Source: CAD feature listing. Evaluate the final solid. Frame: model axes, mm. Face numbers are marked on the shaded views. Round coordinates to 2 decimals unless told otherwise and drop trailing zeros. Loops run counter-clockwise (first coordinate to the right, second up) from the corner with the lowest first, then second, coordinate; pieces in that order, holes last.
(1) Section C-C, the plane y = 0. Return the cut outline in (x, z), plus the area to 3 significant figures.
(2) Section B-B, the plane x = -20. Return the cut outline in (y, z), plus the area to 3 significant figures.
(3) Material intervals for probe 1 along X at (y, z) = (-3.75, -6.35); probe 2 along Z at (x, y) = (4, 1); probe 3 along X at (y, z) = (-0.25, -2), sorted ascending.
(4) Section D-D, the plane x = 35. Return the cut outline in (y, z), plus the area to 3 significant figures.
(5) Section A-A, the plane z = -6.35. Return the cut outline in (x, y).
(6) First-contact query: pin 1 Ø3 at (x, y) = (-35, 0) entering from -Z; pin 2 Ø4 at (x, y) = (-14.5, 2.5) entering from +Z. Flat tips, straight axial feed; report the tip coordinate or a pass-through.
(7) Mould query, pull axis Z, two halves, no side actions, for the marked faces 1, 2 and 3. Classes: pulls with the +Z half, pulls with the -Z half, needs draft (parallel to the pull), parting line crosses it, or undercut.
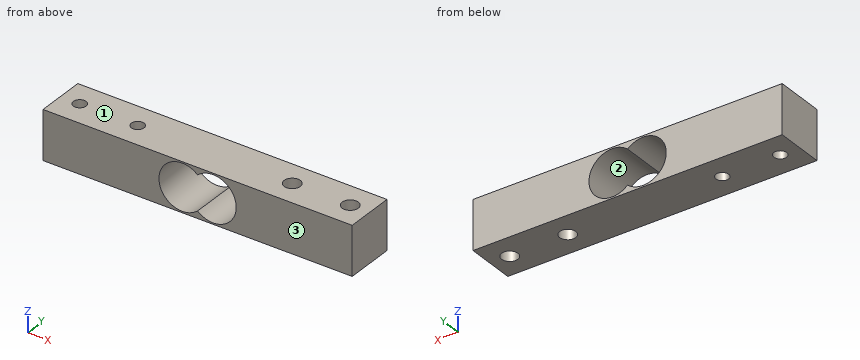
```python
from build123d import *

# Parameters (mm, degrees)
SKETCH1_W               = 80
SKETCH1_H               = 12.7
BOSS_EXTRUDE1_DEPTH     = 12.7
TAP_DRILL_FOR_M5_TAP1_D = 4.2
TAP_DRILL_FOR_M4_TAP1_D = 3.3
SKETCH6_R               = 6
CUT_EXTRUDE1_DEPTH      = 44.847234804


with BuildPart() as part:
    # Sketch1 → Boss-Extrude1 (new body)
    with BuildSketch(Plane.XY):
        Rectangle(SKETCH1_W, SKETCH1_H)
    extrude(amount=-BOSS_EXTRUDE1_DEPTH)

    # Tap Drill for M5 Tap1 (through all)
    with Locations(Plane.XY):
        with Locations((20, 0), (35, 0)):
            Hole(TAP_DRILL_FOR_M5_TAP1_D / 2)

    # Tap Drill for M4 Tap1 (through all)
    with Locations(Plane.XY):
        with Locations((-35, 0), (-20, 0)):
            Hole(TAP_DRILL_FOR_M4_TAP1_D / 2)

    # Sketch6 → Cut-Extrude1 (cut, through all)
    with BuildSketch(Plane(origin=(0, 6.35, 0), x_dir=(1, 0, 0), z_dir=(0, 1, 0))):
        with Locations((-4, 6.35)):
            Circle(SKETCH6_R)
        with Locations((4, 6.35)):
            Circle(SKETCH6_R)
    extrude(amount=-CUT_EXTRUDE1_DEPTH, mode=Mode.SUBTRACT)


solid = part.part
```
Output values:
1. outline: (-40, -12.7) - (-36.65, -12.7) - (-36.65, 0) - (-40, 0) - close; (-33.35, -12.7) - (-21.65, -12.7) - (-21.65, 0) - (-33.35, 0) - close; (-18.35, -12.7) - (17.9, -12.7) - (17.9, 0) - (-18.35, 0) - close; (22.1, -12.7) - (32.9, -12.7) - (32.9, 0) - (22.1, 0) - close; (37.1, -12.7) - (40, -12.7) - (40, 0) - (37.1, 0) - close; hole (0, -10.82) arc R6 ccw (long way) to (0, -1.88) arc R6 ccw (long way) to start
1. area: 624 mm2
2. outline: (-6.35, -12.7) - (-1.65, -12.7) - (-1.65, 0) - (-6.35, 0) - close; (1.65, -12.7) - (6.35, -12.7) - (6.35, 0) - (1.65, 0) - close
2. area: 119 mm2
3. probe 1: x = -40 to -10, 10 to 40
3. probe 2: z = -12.7 to -12.35, -0.35 to 0
3. probe 3: x = -40 to -36.63, -33.37 to -21.63, -18.37 to -8.13, 8.13 to 17.91, 22.09 to 32.91, 37.09 to 40
4. outline: (-6.35, -12.7) - (-2.1, -12.7) - (-2.1, 0) - (-6.35, 0) - close; (2.1, -12.7) - (6.35, -12.7) - (6.35, 0) - (2.1, 0) - close
4. area: 108 mm2
5. outline: (-40, -6.35) - (-10, -6.35) - (-10, 6.35) - (-40, 6.35) - close; (10, -6.35) - (40, -6.35) - (40, 6.35) - (10, 6.35) - close; hole circle Ø3.3 at (-35, 0); hole circle Ø3.3 at (-20, 0); hole circle Ø4.2 at (20, 0); hole circle Ø4.2 at (35, 0)
6. pin 1: passes through
6. pin 2: stops at z = 0
7. face 1: pulls with the +Z half
7. face 2: undercut
7. face 3: needs draft
